Autodesk Inventor part; units mm, degrees
ref_plane "YZ Plane" through (0, 0, 0) normal (1, 0, 0) x (0, 1, 0)
ref_plane "XZ Plane" through (0, 0, 0) normal (0, 1, 0) x (-1, 0, 0)
ref_plane "XY Plane" through (0, 0, 0) normal (0, 0, 1) x (1, 0, 0)
sketch "Sketch1" plane through (0, 0, 0) normal (0, 0, 1) x (1, 0, 0)
  circle A0 centre (0, 0) radius 150 construction
  line L0 (0, -150) -> (-129.9038, -75)
  line L1 (-129.9038, -75) -> (-129.9038, 75)
  line L2 (-129.9038, 75) -> (0, 150)
  line L3 (0, 150) -> (129.9038, 75)
  line L4 (129.9038, 75) -> (129.9038, -75)
  line L5 (129.9038, -75) -> (0, -150)
  circle A1 centre (0, 0) radius 6.154 construction
  line L6 (30, 0) -> (15, -25.9808) construction
  line L7 (15, -25.9808) -> (-15, -25.9808) construction
  line L8 (-15, -25.9808) -> (-30, 0) construction
  line L9 (-30, 0) -> (-15, 25.9808) construction
  line L10 (-15, 25.9808) -> (15, 25.9808) construction
  line L11 (15, 25.9808) -> (30, 0) construction
  line L12 (-129.9038, 57.6795) -> (-114.9038, 83.6603)
  line L13 (-15, 141.3397) -> (15, 141.3397)
  line L14 (129.9038, 57.6795) -> (114.9038, 83.6603)
  line L15 (129.9038, -57.6795) -> (114.9038, -83.6603)
  line L16 (-15, -141.3397) -> (15, -141.3397)
  line L17 (-129.9038, -57.6795) -> (-114.9038, -83.6603)
  line L18 (-129.9038, 75) -> (129.9038, -75) construction
  line L19 (-125.9038, 81.9282) -> (133.9038, -68.0718) construction
  line L20 (-133.9038, 68.0718) -> (125.9038, -81.9282) construction
  line L21 (-125.5737, 55.1795) -> (-110.5737, 81.1603) construction
  circle A2 centre (-114.0737, 75.0981) radius 1.1
  circle A3 centre (-122.0737, 61.2417) radius 1.1
  line L22 (-133.9038, -68.0718) -> (125.9038, 81.9282) construction
  line L23 (-129.9038, -75) -> (129.9038, 75) construction
  line L24 (-125.9038, -81.9282) -> (133.9038, 68.0718) construction
  line L25 (-110.5737, -81.1603) -> (-125.5737, -55.1795) construction
  circle A4 centre (-114.0737, -75.0981) radius 1.1
  circle A5 centre (-122.0737, -61.2417) radius 1.1
  line L26 (-8, -150) -> (-8, 150) construction
  line L27 (0, -150) -> (0, 150) construction
  line L28 (8, -150) -> (8, 150) construction
  line L29 (15, -136.3397) -> (-15, -136.3397) construction
  circle A6 centre (8, -136.3397) radius 1.1
  circle A7 centre (-8, -136.3397) radius 1.1
  line L30 (125.9038, -81.9282) -> (-133.9038, 68.0718) construction
  line L31 (129.9038, -75) -> (-129.9038, 75) construction
  line L32 (133.9038, -68.0718) -> (-125.9038, 81.9282) construction
  line L33 (125.5737, -55.1795) -> (110.5737, -81.1603) construction
  circle A8 centre (122.0737, -61.2417) radius 1.1
  circle A9 centre (114.0737, -75.0981) radius 1.1
  line L34 (133.9038, 68.0718) -> (-125.9038, -81.9282) construction
  line L35 (129.9038, 75) -> (-129.9038, -75) construction
  line L36 (125.9038, 81.9282) -> (-133.9038, -68.0718) construction
  line L37 (110.5737, 81.1603) -> (125.5737, 55.1795) construction
  circle A10 centre (114.0737, 75.0981) radius 1.1
  circle A11 centre (122.0737, 61.2417) radius 1.1
  line L38 (8, 150) -> (8, -150) construction
  line L39 (0, 150) -> (0, -150) construction
  line L40 (-8, 150) -> (-8, -150) construction
  line L41 (-15, 136.3397) -> (15, 136.3397) construction
  circle A12 centre (-8, 136.3397) radius 1.1
  circle A13 centre (8, 136.3397) radius 1.1
  dimension "d5" = 300
  dimension "d6" = 30
  dimension "d7" = 30
  dimension "d8" = 30
  dimension "d9" = 30
  dimension "d10" = 30
  dimension "d11" = 30
  dimension "d12" = 30
  dimension "d17" = 8
  dimension "d18" = 8
  dimension "d19" = 5
  dimension "d20" = 2.2
  dimension "d21" = 2.2
  dimension "d24" = 360
extrude "Extrusion1" add sketch "Sketch1" along normal blind 3.5 contours L0 L17 L1 L12 L2 L13 L3 L14 L4 L15 L5 L16
properties part number "Body_Plate"
The listing builds one solid part. Answer for the finished solid, in the listing's coordinates (mm). Coordinates: 2 decimals unless noted, no trailing zeros. Loops run counter-clockwise (first coordinate to the right, second up) from the corner with the lowest first, then second, coordinate; pieces in that order, holes last. Notation, with made-up numbers: (81.5, 66) -> (103.5, 66) arc R26 cw to (103.5, 105) -> close; hole circle Ø5 at (70.25, 37.25). An arc over 180 degrees is marked (long way). Answer in a Markdown table with one row per item. Add a question column.
1. The part is cut by section B-B, the plane x = -107.5. Write down the section's boundary in (y, z), then the cut area to 3 significant figures.
2. The part is cut by section C-C, the plane y = 67.5. Write down the section's boundary in (x, z), then the cut area to 3 significant figures.
3. The part is cut by section A-A, the plane z = 2.9. Count the separate pieces of the cut face and the enclosed holes in it, then the cut area to 3 significant figures.
4. Flat-ended cylindrical pins translate along their axes: P1, Ø1.3, axis at x = -114.07, y = 75.1, coming from the +Z side; P2, Ø3.5, axis at x = -8, y = -136.34, coming from the -Z side; P3, Ø1.5, axis at x = 72.5, z = 2, coming from the -Y side; P4, Ø1, axis at x = -54.5, z = 3, coming from the +Y side. Find the tip coordinate at first contact, or state that the pin passes through.
5. Consider line 1 (Y direction, x = -8, z = 1.5); line 2 (Y direction, x = -8.5, z = 2.75); line 3 (Y direction, x = 30.5, z = 0.55). Determine where each line is inside the solid, lowest interval first. Write a range as [from, to].
Answer below:
| question | item | result |
|---|---|---|
| 1 | outline | (-87.93, 0) -> (87.93, 0) -> (87.93, 3.5) -> (-87.93, 3.5) -> close |
| 1 | area | 616 mm2 |
| 2 | outline | (-124.23, 0) -> (124.23, 0) -> (124.23, 3.5) -> (-124.23, 3.5) -> close |
| 2 | area | 870 mm2 |
| 3 | separate pieces | 1 |
| 3 | enclosed holes | 12 |
| 3 | area | 57,600 mm2 |
| 4 | P1 | through |
| 4 | P2 | z = 0 |
| 4 | P3 | y = -108.58 |
| 4 | P4 | y = 118.82 |
| 5 | line 1 | [-141.34, -137.44], [-135.24, 135.24], [137.44, 141.34] |
| 5 | line 2 | [-141.34, -137.32], [-135.36, 135.36], [137.32, 141.34] |
| 5 | line 3 | [-132.39, 132.39] |
